Here's how the part is built. I have some questions about the finished solid (model axes, mm). Round coordinates to 2 decimals unless told otherwise and drop trailing zeros. Write each loop counter-clockwise with the first axis right and the second up, starting at its lowest first coordinate (ties: lowest second). Pieces come first, ordered by that corner, then holes. Notation, with made-up numbers: (28, 55.25) -> (53, 55.25) arc R8 cw to (53, 68.25) -> close; hole circle Ø8 at (63.5, 62.25). An arc over 180 degrees is marked (long way). Answer as CSV lines item,"result".
from build123d import *

# Parameters (mm, degrees)
BOSS_EXTRUDE1_DEPTH  = 3
CUT_EXTRUDE1_DEPTH   = 3
LPATTERN1_COUNT      = 8
LPATTERN1_PITCH      = 25
MIRROR1_COPY_1_DEPTH = 3
MIRROR1_COPY_2_DEPTH = 3
MIRROR1_COPY_3_DEPTH = 3
MIRROR1_COPY_4_DEPTH = 3
MIRROR1_COPY_5_DEPTH = 3
MIRROR1_COPY_6_DEPTH = 3
MIRROR1_COPY_7_DEPTH = 3
CUT_EXTRUDE3_START   = -3
CUT_EXTRUDE3_DEPTH   = 236.905459961
LPATTERN2_COUNT      = 15
LPATTERN2_PITCH      = 21
CUT_EXTRUDE5_START   = -3
CUT_EXTRUDE5_DEPTH   = 236.905459961
LPATTERN3_COUNT      = 10
LPATTERN3_PITCH      = 21


with BuildPart() as part:
    # Sketch2 → Boss-Extrude1 (new body)
    with BuildSketch(Plane.XY):
        Polygon((-111.410161514, 164.35009364), (111.410161514, 164.35009364), (165, -42.705142442), (-165, -42.705142442), align=None)
    extrude(amount=BOSS_EXTRUDE1_DEPTH)

    # Sketch3 → Cut-Extrude1 (cut)
    with BuildSketch(Plane(origin=(0, 0, 0), x_dir=(-1, 0, 0), z_dir=(0, 0, -1))):
        Polygon((-161.241557894, -28.183637254), (-158.337256856, -28.935325675), (-155.831628785, -19.254322216), (-158.735929823, -18.502633795), align=None)
    cut_extrude1 = extrude(amount=-CUT_EXTRUDE1_DEPTH, mode=Mode.SUBTRACT)

    # LPattern1: Cut-Extrude1 ×8
    with Locations(*[Vector(-0.25056280708573136, 0.9681003458863748, 0) * (i * LPATTERN1_PITCH) for i in range(1, LPATTERN1_COUNT)]):
        add(cut_extrude1, mode=Mode.SUBTRACT)

    # Mirror1: Cut-Extrude1 across plane
    add(cut_extrude1.mirror(Plane(origin=(0, 0, 0), x_dir=(0, 0, 1), z_dir=(1, 0, 0))), mode=Mode.SUBTRACT)

    # Mirror1 copy 1 sketch → Mirror1 copy 1 (cut)
    with BuildSketch(Plane(origin=(6.264070177, 24.202508647, 0), x_dir=(1, 0, 0), z_dir=(0, 0, -1))):
        Polygon((-161.241557894, 28.183637254), (-158.337256856, 28.935325675), (-155.831628785, 19.254322216), (-158.735929823, 18.502633795), align=None)
    extrude(amount=-MIRROR1_COPY_1_DEPTH, mode=Mode.SUBTRACT)

    # Mirror1 copy 2 sketch → Mirror1 copy 2 (cut)
    with BuildSketch(Plane(origin=(12.528140354, 48.405017294, 0), x_dir=(1, 0, 0), z_dir=(0, 0, -1))):
        Polygon((-161.241557894, 28.183637254), (-158.337256856, 28.935325675), (-155.831628785, 19.254322216), (-158.735929823, 18.502633795), align=None)
    extrude(amount=-MIRROR1_COPY_2_DEPTH, mode=Mode.SUBTRACT)

    # Mirror1 copy 3 sketch → Mirror1 copy 3 (cut)
    with BuildSketch(Plane(origin=(18.792210531, 72.607525941, 0), x_dir=(1, 0, 0), z_dir=(0, 0, -1))):
        Polygon((-161.241557894, 28.183637254), (-158.337256856, 28.935325675), (-155.831628785, 19.254322216), (-158.735929823, 18.502633795), align=None)
    extrude(amount=-MIRROR1_COPY_3_DEPTH, mode=Mode.SUBTRACT)

    # Mirror1 copy 4 sketch → Mirror1 copy 4 (cut)
    with BuildSketch(Plane(origin=(25.056280709, 96.810034589, 0), x_dir=(1, 0, 0), z_dir=(0, 0, -1))):
        Polygon((-161.241557894, 28.183637254), (-158.337256856, 28.935325675), (-155.831628785, 19.254322216), (-158.735929823, 18.502633795), align=None)
    extrude(amount=-MIRROR1_COPY_4_DEPTH, mode=Mode.SUBTRACT)

    # Mirror1 copy 5 sketch → Mirror1 copy 5 (cut)
    with BuildSketch(Plane(origin=(31.320350886, 121.012543236, 0), x_dir=(1, 0, 0), z_dir=(0, 0, -1))):
        Polygon((-161.241557894, 28.183637254), (-158.337256856, 28.935325675), (-155.831628785, 19.254322216), (-158.735929823, 18.502633795), align=None)
    extrude(amount=-MIRROR1_COPY_5_DEPTH, mode=Mode.SUBTRACT)

    # Mirror1 copy 6 sketch → Mirror1 copy 6 (cut)
    with BuildSketch(Plane(origin=(37.584421063, 145.215051883, 0), x_dir=(1, 0, 0), z_dir=(0, 0, -1))):
        Polygon((-161.241557894, 28.183637254), (-158.337256856, 28.935325675), (-155.831628785, 19.254322216), (-158.735929823, 18.502633795), align=None)
    extrude(amount=-MIRROR1_COPY_6_DEPTH, mode=Mode.SUBTRACT)

    # Mirror1 copy 7 sketch → Mirror1 copy 7 (cut)
    with BuildSketch(Plane(origin=(43.84849124, 169.41756053, 0), x_dir=(1, 0, 0), z_dir=(0, 0, -1))):
        Polygon((-161.241557894, 28.183637254), (-158.337256856, 28.935325675), (-155.831628785, 19.254322216), (-158.735929823, 18.502633795), align=None)
    extrude(amount=-MIRROR1_COPY_7_DEPTH, mode=Mode.SUBTRACT)

    # Sketch4 → Cut-Extrude3 (cut)
    with BuildSketch(Plane(origin=(0, 0, 0), x_dir=(-1, 0, 0), z_dir=(0, 0, -1)).offset(CUT_EXTRUDE3_START)):
        Polygon((-154, -813.317713437), (-154, -42.705142442), (-154, -32.705142442), (-144, -32.705142442), (-144, -42.705142442), (-144, -813.317713437), (-144, -2354.542855427), (-154, -2354.542855427), align=None)
    cut_extrude3 = extrude(amount=CUT_EXTRUDE3_DEPTH, mode=Mode.SUBTRACT)

    # LPattern2: Cut-Extrude3 ×15
    with Locations(*[(-i * LPATTERN2_PITCH, 0, 0) for i in range(1, LPATTERN2_COUNT)]):
        add(cut_extrude3, mode=Mode.SUBTRACT)

    # Sketch5 → Cut-Extrude5 (cut)
    with BuildSketch(Plane(origin=(0, 0, 0), x_dir=(-1, 0, 0), z_dir=(0, 0, -1)).offset(CUT_EXTRUDE5_START)):
        Polygon((-100.410161514, 847.594253284), (-100.410161514, 164.35009364), (-100.410161514, 161.35009364), (-90.410161514, 161.35009364), (-90.410161514, 164.35009364), (-90.410161514, 847.594253284), (-90.410161514, 2214.082572573), (-100.410161514, 2214.082572573), align=None)
    cut_extrude5 = extrude(amount=CUT_EXTRUDE5_DEPTH, mode=Mode.SUBTRACT)

    # LPattern3: Cut-Extrude5 ×10
    with Locations(*[(-i * LPATTERN3_PITCH, 0, 0) for i in range(1, LPATTERN3_COUNT)]):
        add(cut_extrude5, mode=Mode.SUBTRACT)


solid = part.part
Item 1: Suppose I cut it at B-B, the plane y = -14. List the corners of the cut face in (x, z) for me.
Results found:
outline,"(-157.57, 0) -> (157.57, 0) -> (157.57, 3) -> (-157.57, 3) -> close"
Item 2: I need wall thicknesses on L1, parallel to Y at x = 107, z = 1.45; L2, parallel to Y at x = 71.5, z = 1.3; L3, parallel to X at y = 84, z = 2.05. Which ranges of each line are inside material? Lowest first, please.
Results found:
L1,"y = -32.71 to 164.35"
L2,"y = -42.71 to 161.35"
L3,"x = -132.21 to 132.21"
Item 3: Will these pins go through, and if not, where does the flat tip stop? pin 1 (1.5 mm diameter, centred on x = -101.5, z = 1.5, fed in from -Y); pin 2 (0.9 mm diameter, centred on y = 162.5, z = 1.5, fed in from -X); pin 3 (0.9 mm diameter, centred on y = -35.5, z = 2, fed in from -X).
Results found:
pin 1,"stops at y = -32.71"
pin 2,"stops at x = -112.01"
pin 3,"stops at x = -163.25"
Item 4: Suppose I cut it at A-A, the plane x = 105.5. List the corners of the cut face in (y, z) for me, then the cut area to 3 significant figures.
Results found:
outline,"(-32.71, 0) -> (164.35, 0) -> (164.35, 3) -> (-32.71, 3) -> close"
area,"591 mm²"
